Here's how the part is built. I have some questions about the finished solid (model axes, mm). A direction names the side the tool comes from. Coordinates: 2 decimals unless noted, no trailing zeros. Loops run counter-clockwise (first coordinate to the right, second up) from the corner with the lowest first, then second, coordinate; pieces in that order, holes last. Notation, with made-up numbers: (21.25, -21) -> (75.25, -21) arc R17 cw to (75.25, -1) -> close; hole circle Ø1 at (67.5, -23). An arc over 180 degrees is marked (long way). Answer as a JSON object with one key per item and string values. Group by question number.
1) I'm going to push flat-ended pins straight in: pin 1 (7 mm diameter, centred on y = 51.5, z = 50.5, fed in from -X); pin 2 (3 mm diameter, centred on x = -438.5, y = 32, fed in from -Z); pin 3 (6 mm diameter, centred on y = 9, z = 341.5, fed in from +X); pin 4 (2 mm diameter, centred on x = -317, z = 326.5, fed in from -Y). Where does each tip first touch, or does it pass through?
2) I need wall thicknesses on probe 1 along Y at (x, z) = (-447, 0); probe 2 along Z at (x, y) = (-313.5, 54.5); probe 3 along X at (y, z) = (48.5, -386). Which ranges of each line are inside material? Lowest first, please. Write a range as [from, to].
3) If we mould it in two halves opening along X, with no side actions, what happens to faces 1 (the flat face through (446, 39, -45)), 2 (the flat face through (293, 0, -329)), 3 (the cylindrical face through (-478.35, 39.44, -106.22))? For each: +X half, -X half, draft (parallel to the pull), parting line (faces both ways), or undercut.
4) I want a section at C-C (y = 40). Write out the boundary of the cut face in (x, z).
5) I want a section at B-B (z = 0). Write out the boundary of the cut face in (x, y).
6) I want a section at D-D (x = -356.5). Write out the boundary of the cut face in (y, z), then the cut area to 3 significant figures.
7) I want a section at A-A (x = 0). Write out the boundary of the cut face in (y, z).
8) Which directions (+Z, -Z, +X, -X, +Y, -Y) give clear straight access to the entire face, cutting with the end or side of a thin tool? Please do faces 4 (the cylindrical face through (-445.916, 70.736, 4.036)), 5 (the cylindrical face through (8.137, 39.44, -439.925)), 6 (the flat face through (293, 80, -329)).
```python
from build123d import *

# Parameters (mm, degrees)
SKETCH1_R               = 490
SKETCH1_R_2             = 440
BOSS_EXTRUDE1_DEPTH     = 80
CUT_EXTRUDE2_DEPTH      = 698.567201064
CUT_EXTRUDE2_DEPTH_BACK = 698.567201064
SKETCH4_W               = 110
SKETCH4_H               = 80
CUT_EXTRUDE3_DEPTH      = 10
SKETCH5_R               = 31
CUT_EXTRUDE4_DEPTH      = 12


with BuildPart() as part:
    # Sketch1 → Boss-Extrude1 (new body)
    with BuildSketch(Plane(origin=(0, 0, 0), x_dir=(1, 0, 0), z_dir=(0, 1, 0))):
        with Locations(Location((0, 0, 0), (0, 0, 270))):
            Circle(SKETCH1_R)
        with Locations(Location((0, 0, 0), (0, 0, 270))):
            Circle(SKETCH1_R_2, mode=Mode.SUBTRACT)
    extrude(amount=BOSS_EXTRUDE1_DEPTH)

    # Sketch3 → Cut-Extrude2 (cut, two sides: drawn at the far end of the back side and taken through both)
    with BuildSketch(Plane(origin=(0, 80, 0), x_dir=(1, 0, 0), z_dir=(0, 1, 0)).offset(-CUT_EXTRUDE2_DEPTH_BACK)):
        Polygon((446, 32.5), (454, 32.5), (454, -32.5), (446, -32.5), (446, -56.5), (366.03, -56.5), (366.03, 56.5), (446, 56.5), align=None)
    extrude(amount=CUT_EXTRUDE2_DEPTH + CUT_EXTRUDE2_DEPTH_BACK, mode=Mode.SUBTRACT)

    # Sketch4 → Cut-Extrude3 (cut)
    with BuildSketch(Plane(origin=(-440, 0, 0), x_dir=(0, 0, -1), z_dir=(1, 0, 0))):
        with Locations((0, 40)):
            Rectangle(SKETCH4_W, SKETCH4_H)
    extrude(amount=CUT_EXTRUDE3_DEPTH, mode=Mode.SUBTRACT)

    # Sketch5 → Cut-Extrude4 (cut)
    with BuildSketch(Plane(origin=(-440, 0, 0), x_dir=(0, 0, -1), z_dir=(1, 0, 0))):
        with Locations((0, 40)):
            Circle(SKETCH5_R)
    extrude(amount=-CUT_EXTRUDE4_DEPTH, mode=Mode.SUBTRACT)


solid = part.part
```
Determined:
{
 "1": {"pin 1": "x = -487.74", "pin 2": "z = -221.66", "pin 3": "x = 354.28", "pin 4": "y = 0"},
 "2": {"probe 1": "[0, 9], [71, 80]", "probe 2": "[-376.59, -308.74], [308.74, 376.59]", "probe 3": "[-301.83, -211.2], [211.2, 301.83]"},
 "3": {"face 1": "undercut", "face 2": "draft", "face 3": "parting line"},
 "4": {"outline": "circle Ø980 at (0, 0); hole (-452, -31) -> (-440, -31) -> (-440, -55) -> (-436.55, -55) arc R440 ccw to (436.36, -56.5) -> (446, -56.5) -> (446, -32.5) -> (454, -32.5) -> (454, 32.5) -> (446, 32.5) -> (446, 56.5) -> (436.36, 56.5) arc R440 ccw to (-436.55, 55) -> (-440, 55) -> (-440, 31) -> (-452, 31) -> close"},
 "5": {"outline": "(-490, 0) -> (-440, 0) -> (-440, 9) -> (-452, 9) -> (-452, 71) -> (-440, 71) -> (-440, 80) -> (-490, 80) -> close; (454, 0) -> (490, 0) -> (490, 80) -> (454, 80) -> close"},
 "6": {"outline": "(0, -336.17) -> (80, -336.17) -> (80, -257.89) -> (0, -257.89) -> close; (0, 257.89) -> (80, 257.89) -> (80, 336.17) -> (0, 336.17) -> close", "area": "12,500 mm^2"},
 "7": {"outline": "(0, -490) -> (80, -490) -> (80, -440) -> (0, -440) -> close; (0, 440) -> (80, 440) -> (80, 490) -> (0, 490) -> close"},
 "8": {"face 4": "none", "face 5": "+Y, -Y", "face 6": "+Z, -Z, +X, -X, +Y"}
}
